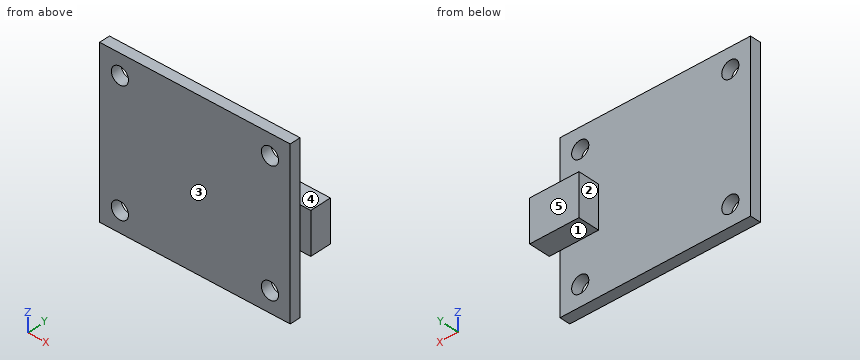
from build123d import *

# Parameters (mm, degrees)
SKETCH1_W           = 35.56
SKETCH1_H           = 30.51
BOSS_EXTRUDE1_DEPTH = 2
SKETCH2_R           = 1.6
CUT_EXTRUDE1_DEPTH  = 24.512622674
SKETCH3_W           = 9.2
SKETCH3_H           = 7.8
BOSS_EXTRUDE2_DEPTH = 4


with BuildPart() as part:
    # Sketch1 → Boss-Extrude1 (new body)
    with BuildSketch(Plane(origin=(0, 0, 0), x_dir=(1, 0, 0), z_dir=(0, 1, 0))):
        Rectangle(SKETCH1_W, SKETCH1_H)
    extrude(amount=BOSS_EXTRUDE1_DEPTH)

    # Sketch2 → Cut-Extrude1 (cut, through all)
    with BuildSketch(Plane(origin=(0, 2, 0), x_dir=(1, 0, 0), z_dir=(0, 1, 0))):
        with Locations(Location((-14, 11.425, 0), (0, 0, 270))):
            Circle(SKETCH2_R)
        with Locations(Location((14, 11.425, 0), (0, 0, 270))):
            Circle(SKETCH2_R)
        with Locations(Location((14, -11.425, 0), (0, 0, 270))):
            Circle(SKETCH2_R)
        with Locations(Location((-14, -11.425, 0), (0, 0, 270))):
            Circle(SKETCH2_R)
    extrude(amount=-CUT_EXTRUDE1_DEPTH, mode=Mode.SUBTRACT)

    # Sketch3 → Boss-Extrude2 (add)
    with BuildSketch(Plane(origin=(0, 2, 0), x_dir=(1, 0, 0), z_dir=(0, 1, 0))):
        with Locations((15.18, 0)):
            Rectangle(SKETCH3_W, SKETCH3_H)
    extrude(amount=BOSS_EXTRUDE2_DEPTH)


solid = part.part
Verification items for the finished model (mm, model axes). Face numbers are marked on the shaded views. A direction names the side the tool comes from. Coordinates: 2 decimals unless noted, no trailing zeros. Order: outer loops, then holes, each group sorted by start corner. A loop starts at its lowest first (then second) coordinate and runs counter-clockwise, first axis right, second up. Notation, with made-up numbers: M -23.75,-21.75 L 15.25,-21.75 A27 ccw 15.25,11.25 Z; hole C -8,-31 d4. An arc over 180 degrees is marked long. Write each question's results on one line, items separated by ' | '.
1) Section check A-A on x = 14. Record the cut outline in (y, z) (3 decimals), plus the area to 3 significant figures.
Solved:
outline: M 0,-15.255 L 2,-15.255 L 2,-13.025 L 0,-13.025 Z; M 0,-9.825 L 2,-9.825 L 2,-3.9 L 6,-3.9 L 6,3.9 L 2,3.9 L 2,9.825 L 0,9.825 Z; M 0,13.025 L 2,13.025 L 2,15.255 L 0,15.255 Z | area: 79.4 mm²
2) Section check D-D on x = -14. Record the cut outline in (y, z) (3 decimals), plus the area to 3 significant figures.
Solved:
outline: M 0,-15.255 L 2,-15.255 L 2,-13.025 L 0,-13.025 Z; M 0,-9.825 L 2,-9.825 L 2,9.825 L 0,9.825 Z; M 0,13.025 L 2,13.025 L 2,15.255 L 0,15.255 Z | area: 48.2 mm²
3) Scan lines: line 1 along X through (y, z) = (1.7, -10.5); line 2 along Y through (x, z) = (18.5, 0.5); line 3 along Y through (x, z) = (-15, -7). Record each from-to range of solid material in increasing order. Write a range as [from, to].
Solved:
line 1: x = [-17.78, -15.31], [-12.69, 12.69], [15.31, 17.78] | line 2: y = [2, 6] | line 3: y = [0, 2]
4) Access from +Z, -Z, +X, -X, +Y, -Y to the whole of each face (thin tool, end or side, straight path). Record for the marked faces 1, 2, 3, 4 and 5.
Solved:
face 1: -Z, +X, -X, +Y | face 2: +Z, -Z, -X, +Y | face 3: +Z, -Z, +X, -X, -Y | face 4: +Z, +X, -X, +Y | face 5: +Z, -Z, +X, -X, +Y
5) Section check B-B on y = 1.1. Record the cut outline in (x, z) (3 decimals).
Solved:
outline: M -17.78,-15.255 L 17.78,-15.255 L 17.78,15.255 L -17.78,15.255 Z; hole C -14,-11.425 d3.2; hole C -14,11.425 d3.2; hole C 14,-11.425 d3.2; hole C 14,11.425 d3.2
6) Section check C-C on z = 12. Record the cut outline in (x, y).
Solved:
outline: M -17.78,0 L -15.49,0 L -15.49,2 L -17.78,2 Z; M -12.51,0 L 12.51,0 L 12.51,2 L -12.51,2 Z; M 15.49,0 L 17.78,0 L 17.78,2 L 15.49,2 Z
7) Gauge pin test, flat ends, axial feed: pin 1 Ø3 at (x, y) = (16, 5) entering from +Z; pin 2 Ø2 at (y, z) = (1, 7) entering from +X; pin 3 Ø1.6 at (x, z) = (19, 0) entering from -Y; pin 4 Ø2 at (x, y) = (11, 2.5) entering from +Z (3 decimals). Record the tip position at first contact, or that the pin passes through.
Solved:
pin 1: stops at z = 3.9 | pin 2: stops at x = 17.78 | pin 3: stops at y = 2 | pin 4: stops at z = 15.255
